```python
from build123d import *

# Parameters (mm, degrees)
F0_W     = 47.625
F0_H     = 47.625
F1_DEPTH = 77.7875
F2_W     = 50.8
F2_H     = 50.8
F3_DEPTH = 3.175


with BuildPart() as f1:
    # F0 (on Right) → F1 (new body)
    with BuildSketch(Plane.YZ):
        Rectangle(F0_W, F0_H)
    extrude(amount=F1_DEPTH)

    # F2 (on face) → F3 (join)
    with BuildSketch(Plane.YZ.offset(77.7875)):
        Rectangle(F2_W, F2_H)
    extrude(amount=F3_DEPTH)


solid = f1.part
```
Geometry check sheet. Reference: the model listing, model coordinates, mm. A direction names the side the tool comes from. Coordinates: 2 decimals unless noted, no trailing zeros. Loops run counter-clockwise (first coordinate to the right, second up) from the corner with the lowest first, then second, coordinate; pieces in that order, holes last. Notation, with made-up numbers: (20, 82) -> (55, 82) arc R16 cw to (55, 93) -> close; hole circle Ø8 at (84, 8.25). An arc over 180 degrees is marked (long way). Put each result on its own line as item: value.
1) Tool access check on faces 1 (the flat face through (79, 0, -25.4)), 2 (the flat face through (38, 0, 23.812)), 3 (the flat face through (38, 23.812, 0)), 4 (the flat face through (38, -23.812, 0)), 5 (the flat face through (38, 0, -23.812)). Record the directions out of +Z, -Z, +X, -X, +Y, -Y that give a thin tool (end or side, any length) a straight path to the whole face; none if there is none.
Result set:
face 1: -Z, +X, -X, +Y, -Y
face 2: +Z, -X, +Y, -Y
face 3: +Z, -Z, -X, +Y
face 4: +Z, -Z, -X, -Y
face 5: -Z, -X, +Y, -Y
2) Cross-section at A-A on z = 11.5. Record the boundary of the cut face in (x, y).
Result set:
outline: (0, -23.81) -> (77.79, -23.81) -> (77.79, -25.4) -> (80.96, -25.4) -> (80.96, 25.4) -> (77.79, 25.4) -> (77.79, 23.81) -> (0, 23.81) -> close
3) Cross-section at C-C on x = 35. Record the boundary of the cut face in (y, z).
Result set:
outline: (-23.81, -23.81) -> (23.81, -23.81) -> (23.81, 23.81) -> (-23.81, 23.81) -> close
4) Gauge pin test, flat ends, axial feed: pin 1 Ø3 at (x, y) = (58.5, -18) entering from -Z; pin 2 Ø8 at (x, z) = (56, 0.5) entering from -Y; pin 3 Ø24 at (x, z) = (53, 10) entering from +Y; pin 4 Ø3 at (y, z) = (15, -8.5) entering from -X. Record the tip position at first contact, or that the pin passes through.
Result set:
pin 1: stops at z = -23.81
pin 2: stops at y = -23.81
pin 3: stops at y = 23.81
pin 4: stops at x = 0
5) Thickness scan on line 1 (Y direction, x = 33.5, z = 18.5). Record the ranges inside material, lowest first.
Result set:
line 1: y = -23.81 to 23.81
